Check sheet for the modelled part. Datum: model origin and axes. Units: mm. Face numbers are marked on the shaded views. Coordinates: 2 decimals unless noted, no trailing zeros. Loops run counter-clockwise (first coordinate to the right, second up) from the corner with the lowest first, then second, coordinate; pieces in that order, holes last. Notation, with made-up numbers: (-30.75, 34) - (-20.75, 34) arc R23 ccw to (-20.75, 62) - close; hole circle Ø6 at (83.5, -20). An arc over 180 degrees is marked (long way). Use a Markdown table: item, result. Add a question column.
1) Sectioned sample at A-A, the plane z = 1.15. Enter the section's corners in (x, y), then the cut area to 3 significant figures.
2) Go/stop test with flat-tipped pins: P1, Ø1, axis at x = -9, z = 2.5, coming from the +Y side; P2, Ø1.5, axis at x = 9.5, y = 2.5, coming from the -Z side; P3, Ø1, axis at y = 6.5, z = 2, coming from the -X side; P4, Ø1.5, axis at y = -20.5, z = 2, coming from the +X side. Record where each tip stops, or that it passes through.
3) Sectioned sample at D-D, the plane y = 0. Enter the section's corners in (x, z).
4) Draft check along Y on the marked faces 1, 2 and 3. Enter one of: pulls with the +Y half, pulls with the -Y half, needs draft (parallel to the pull), parting line crosses it, or undercut.
5) Thickness scan on line 1 (Y direction, x = 0, z = 2.4); line 2 (Y direction, x = -15, z = 0.6); line 3 (X direction, y = -17, z = 2.4). Record the ranges inside material, lowest first.
6) Sectioned sample at C-C, the plane y = -19. Enter the section's corners in (x, z), then the cut area to 3 significant figures.
7) Sectioned sample at B-B, the plane x = 0. Enter the section's corners in (y, z).
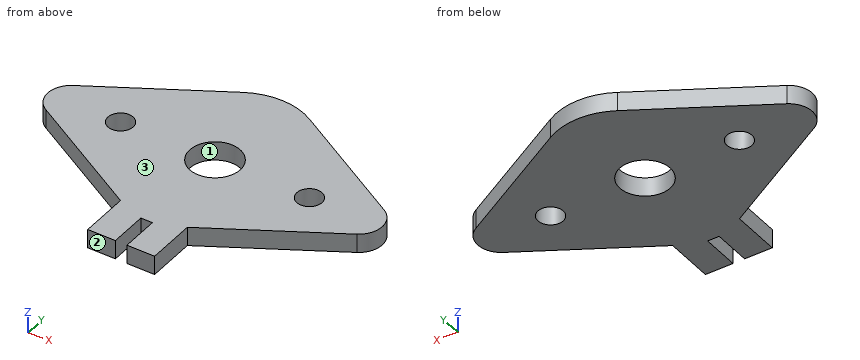
from build123d import *

# Parameters (mm, degrees)
SKETCH_1_R      = 4
SKETCH_1_R_2    = 2
EXTRUDE_1_DEPTH = 3


with BuildPart() as part:
    # 草图1 → 凸台-拉伸1 (new body)
    with BuildSketch(Plane.XY):
        with BuildLine():
            Line((5.309266756, 14.424138209), (24.693114579, 3.23286845))
            ThreePointArc((24.693114579, 3.23286845), (26.559612049, 0), (24.693114579, -3.23286845))
            Line((24.693114579, -3.23286845), (5.309266756, -14.424138209))
            Line((5.309266756, -14.424138209), (5.309266756, -22.162123177))
            Line((5.309266756, -22.162123177), (0.916263641, -22.162123177))
            Line((0.916263641, -22.162123177), (0.916263641, -16.150751559))
            Line((0.916263641, -16.150751559), (-0.916263641, -16.150751559))
            Line((-0.916263641, -16.150751559), (-0.916263641, -22.162123177))
            Line((-0.916263641, -22.162123177), (-5.309266756, -22.162123177))
            Line((-5.309266756, -22.162123177), (-5.309266756, -14.424138209))
            Line((-5.309266756, -14.424138209), (-24.693114579, -3.23286845))
            ThreePointArc((-24.693114579, -3.23286845), (-26.559612049, 0), (-24.693114579, 3.23286845))
            Line((-24.693114579, 3.23286845), (-5.309266756, 14.424138209))
            ThreePointArc((-5.309266756, 14.424138209), (0, 15.846751948), (5.309266756, 14.424138209))
        make_face()
        Circle(SKETCH_1_R, mode=Mode.SUBTRACT)
        with Locations((15, 0)):
            Circle(SKETCH_1_R_2, mode=Mode.SUBTRACT)
        with Locations(Location((-15, 0, 0), (0, 0, 180))):
            Circle(SKETCH_1_R_2, mode=Mode.SUBTRACT)
    extrude(amount=EXTRUDE_1_DEPTH)


solid = part.part
Solved:
| question | item | result |
|---|---|---|
| 1 | outline | (-24.69, -3.23) - (-5.31, -14.42) - (-5.31, -22.16) - (-0.92, -22.16) - (-0.92, -16.15) - (0.92, -16.15) - (0.92, -22.16) - (5.31, -22.16) - (5.31, -14.42) - (24.69, -3.23) arc R3.73 ccw to (24.69, 3.23) - (5.31, 14.42) arc R10.62 ccw to (-5.31, 14.42) - (-24.69, 3.23) arc R3.73 ccw to start; hole circle Ø4 at (-15, 0); hole circle Ø8 at (0, 0); hole circle Ø4 at (15, 0) |
| 1 | area | 1,010 mm2 |
| 2 | P1 | stops at y = 12.58 |
| 2 | P2 | stops at z = 0 |
| 2 | P3 | stops at x = -19.9 |
| 2 | P4 | stops at x = 5.31 |
| 3 | outline | (-26.56, 0) - (-17, 0) - (-17, 3) - (-26.56, 3) - close; (-13, 0) - (-4, 0) - (-4, 3) - (-13, 3) - close; (4, 0) - (13, 0) - (13, 3) - (4, 3) - close; (17, 0) - (26.56, 0) - (26.56, 3) - (17, 3) - close |
| 4 | face 1 | undercut |
| 4 | face 2 | pulls with the -Y half |
| 4 | face 3 | needs draft |
| 5 | line 1 | y = -16.15 to -4, 4 to 15.85 |
| 5 | line 2 | y = -8.83 to -2, 2 to 8.83 |
| 5 | line 3 | x = -5.31 to -0.92, 0.92 to 5.31 |
| 6 | outline | (-5.31, 0) - (-0.92, 0) - (-0.92, 3) - (-5.31, 3) - close; (0.92, 0) - (5.31, 0) - (5.31, 3) - (0.92, 3) - close |
| 6 | area | 26.4 mm2 |
| 7 | outline | (-16.15, 0) - (-4, 0) - (-4, 3) - (-16.15, 3) - close; (4, 0) - (15.85, 0) - (15.85, 3) - (4, 3) - close |
